from build123d import *

# Parameters (mm, degrees)
F0_R     = 1.1
F1_DEPTH = 1.5
F2_W     = 20
F2_H     = 1.5
F3_DEPTH = 3


with BuildPart() as f1:
    # F0 (on Top) → F1 (new body)
    with BuildSketch(Plane.XY):
        with BuildLine():
            Line((-5.55, -8.5), (16.25, 8.5))
            Line((16.25, 8.5), (-16.25, 8.5))
            Line((-16.25, 8.5), (-16.25, 4))
            Line((-16.25, 4), (-13.75, 4))
            ThreePointArc((-13.75, 4), (-9.75, 0), (-13.75, -4))
            Line((-13.75, -4), (-16.25, -4))
            Line((-16.25, -4), (-16.25, -8.5))
            Line((-16.25, -8.5), (-5.55, -8.5))
        make_face()
        with Locations((-13.75, -6)):
            Circle(F0_R, mode=Mode.SUBTRACT)
        with Locations((-9.507359, -4.242641)):
            Circle(F0_R, mode=Mode.SUBTRACT)
        with Locations((-9.507359, 4.242641)):
            Circle(F0_R, mode=Mode.SUBTRACT)
        with Locations((-7.75, 0)):
            Circle(F0_R, mode=Mode.SUBTRACT)
        with Locations((-13.75, 6)):
            Circle(F0_R, mode=Mode.SUBTRACT)
    extrude(amount=F1_DEPTH)

    # F2 (on face) → F3 (join)
    with BuildSketch(Plane(origin=(0, 8.5, 0), x_dir=(-1, 0, 0), z_dir=(0, 1, 0))):
        with Locations((-6.25, 0.75)):
            Rectangle(F2_W, F2_H)
    extrude(amount=F3_DEPTH)


solid = f1.part
CAD build for the part. Positions are in the model's coordinates, mm. A direction names the side the tool comes from. Round coordinates to 2 decimals unless told otherwise and drop trailing zeros. Write each loop counter-clockwise with the first axis right and the second up, starting at its lowest first coordinate (ties: lowest second). Pieces come first, ordered by that corner, then holes. Notation, with made-up numbers: M -25.75,39 L 7.25,39 A17 cw 7.25,47 Z; hole C -29.5,55 d3. An arc over 180 degrees is marked long. Use a Markdown table: item, result. Add a question column.
1. Flat gauge pin, fed straight in: P1, Ø0.8, axis at x = -14.5, z = 1, coming from the +Y side. Where does the tip first touch, or does it go through?
2. Slice it at B-B on x = -7.75. Give the cut face in (y, z).
3. Slice it at C-C on z = 0.55. Give the cut face in (x, y).
4. Slice it at A-A on y = 0. Give the cut face in (x, z), then the cut area to 4 significant figures.
5. 3-axis set-ups, long thin cutter, end or side, ignore diameter. For faces 4 (the face through (-15, -4, 1)), 5 (the face through (6, 11.5, 1)), 6 (the face through (-10, 8.5, 1)): which of +Z, -Z, +X, -X, +Y, -Y reach the whole face in a straight line?
6. Drill centre lines: probe 1 along Y at (x, z) = (-13.75, 0.5); probe 2 along X at (y, z) = (8.75, 0.95); probe 3 along X at (y, z) = (-7, 0.75). Where is each one in solid material? Low to high.
7. Slice it at D-D on x = -13. Give the cut face in (y, z), then the cut area to 3 significant figures.
8. Pull direction X, two halves, no side cores. Call faces 1 (the face through (-14.85, -5.95, 0.74)), 2 (the face through (-9.75, 0.09, 0.74)), 3 (the face through (-11, -8.5, 1)): released by +X, released by -X, zero draft, split by the parting line, or undercut.
Reply:
| question | item | result |
|---|---|---|
| 1 | P1 | stops at y = 8.5 |
| 2 | outline | M -8.5,0 L -1.1,0 L -1.1,1.5 L -8.5,1.5 Z; M 1.1,0 L 8.5,0 L 8.5,1.5 L 1.1,1.5 Z |
| 3 | outline | M -16.25,-8.5 L -5.55,-8.5 L 16.25,8.5 L 16.25,11.5 L -3.75,11.5 L -3.75,8.5 L -16.25,8.5 L -16.25,4 L -13.75,4 A4 cw -13.75,-4 L -16.25,-4 Z; hole C -13.75,-6 d2.2; hole C -13.75,6 d2.2; hole C -9.51,-4.24 d2.2; hole C -9.51,4.24 d2.2; hole C -7.75,0 d2.2 |
| 4 | outline | M -9.75,0 L -8.85,0 L -8.85,1.5 L -9.75,1.5 Z; M -6.65,0 L 5.35,0 L 5.35,1.5 L -6.65,1.5 Z |
| 4 | area | 19.35 mm^2 |
| 5 | face 4 | +Z, -Z, -X |
| 5 | face 5 | +Z, -Z, +X, -X, +Y |
| 5 | face 6 | +Z, -Z, -X, +Y |
| 6 | probe 1 | y = -8.5 to -7.1, -4.9 to -4, 4 to 4.9, 7.1 to 8.5 |
| 6 | probe 2 | x = -3.75 to 16.25 |
| 6 | probe 3 | x = -16.25 to -14.21, -13.29 to -3.63 |
| 7 | outline | M -8.5,0 L -6.8,0 L -6.8,1.5 L -8.5,1.5 Z; M -5.2,0 L -3.93,0 L -3.93,1.5 L -5.2,1.5 Z; M 3.93,0 L 5.2,0 L 5.2,1.5 L 3.93,1.5 Z; M 6.8,0 L 8.5,0 L 8.5,1.5 L 6.8,1.5 Z |
| 7 | area | 8.88 mm^2 |
| 8 | face 1 | undercut |
| 8 | face 2 | released by -X |
| 8 | face 3 | zero draft |
